For this review, use the dimensioned drawing (mm, ordinates from the lowest corner) and the shaded views. A direction names the side the tool comes from. Coordinates: 2 decimals unless noted, no trailing zeros. Loops run counter-clockwise (first coordinate to the right, second up) from the corner with the lowest first, then second, coordinate; pieces in that order, holes last. Notation, with made-up numbers: (59.5, -13) - (100.5, -13) arc R19 cw to (100.5, -4) - close; hole circle Ø6 at (-30.75, 33). An arc over 180 degrees is marked (long way). Answer in a Markdown table with one row per item. Add a question column.
(1) To check wall thickness, follow L1, parallel to X at y = 17.25, z = 19.5; L2, parallel to X at y = 4, z = 19.5; L3, parallel to Z at x = 7.5, y = 18.75. State the ranges of each line that lie inside material, in increasing order. Write a range as [from, to].
(2) We need section C-C, the plane y = 3. Write out the cut boundary in (x, z), plus the area to 3 significant figures.
(3) We need section B-B, the plane z = 19.5. Write out the cut boundary in (x, y), plus the area to 3 significant figures.
(4) Clearance check with flat-ended pins moving along their axes: pin 1 (5 mm diameter, centred on y = 13, z = 20, fed in from -X); pin 2 (2 mm diameter, centred on x = 35, y = 5, fed in from +Z); pin 3 (4 mm diameter, centred on x = 14, y = 21.5, fed in from -Z); pin 4 (3.5 mm diameter, centred on x = 7.5, z = 19.5, fed in from +Y). State where each tip first meets the part, or that it passes through.
(5) We need section A-A, the plane x = 31.5. Write out the cut boundary in (y, z).
(6) We need section D-D, the plane z = 5.5. Write out the cut boundary in (x, y).
(7) For the marked faces 1 and 2, list the 3-axis set-ups (+Z, -Z, +X, -X, +Y, -Y) from which the entire face can be reached by the end or side of a thin tool; tool diameter is ignored.
(8) The part is to be moulded in two halves that separate along Z. For the marked faces 3, 4 and 5, say which applies: released by +Z, released by -Z, zero draft, split by the parting line, or undercut.
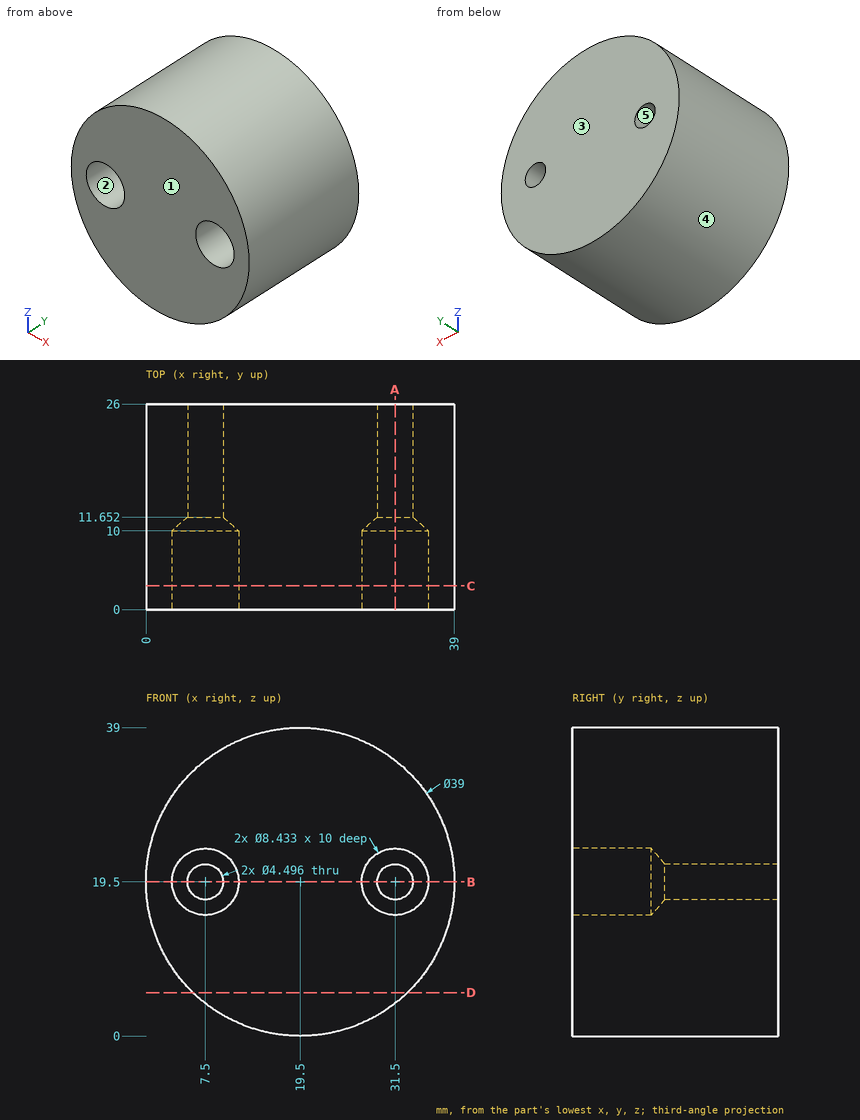
Responses:
| question | item | result |
|---|---|---|
| 1 | L1 | x = [0, 5.25], [9.75, 29.25], [33.75, 39] |
| 1 | L2 | x = [0, 3.28], [11.72, 27.28], [35.72, 39] |
| 1 | L3 | z = [4.13, 17.25], [21.75, 34.87] |
| 2 | outline | circle Ø39 at (19.5, 19.5); hole circle Ø8.43 at (7.5, 19.5); hole circle Ø8.43 at (31.5, 19.5) |
| 2 | area | 1,080 mm2 |
| 3 | outline | (0, 0) - (3.28, 0) - (3.28, 10) - (5.25, 11.65) - (5.25, 26) - (0, 26) - close; (9.75, 11.65) - (11.72, 10) - (11.72, 0) - (27.28, 0) - (27.28, 10) - (29.25, 11.65) - (29.25, 26) - (9.75, 26) - close; (33.75, 11.65) - (35.72, 10) - (35.72, 0) - (39, 0) - (39, 26) - (33.75, 26) - close |
| 3 | area | 695 mm2 |
| 4 | pin 1 | stops at x = 0 |
| 4 | pin 2 | stops at z = 32.54 |
| 4 | pin 3 | stops at z = 0.32 |
| 4 | pin 4 | passes through |
| 5 | outline | (0, 4.13) - (26, 4.13) - (26, 17.25) - (11.65, 17.25) - (10, 15.28) - (0, 15.28) - close; (0, 23.72) - (10, 23.72) - (11.65, 21.75) - (26, 21.75) - (26, 34.87) - (0, 34.87) - close |
| 6 | outline | (5.93, 0) - (33.07, 0) - (33.07, 26) - (5.93, 26) - close |
| 7 | face 1 | +Z, -Z, +X, -X, -Y |
| 7 | face 2 | -Y |
| 8 | face 3 | zero draft |
| 8 | face 4 | split by the parting line |
| 8 | face 5 | undercut |
